The listing builds one solid part. Answer for the finished solid, in the listing's coordinates (mm). Face numbers are marked on the shaded views. A direction names the side the tool comes from. Coordinates: 2 decimals unless noted, no trailing zeros. Order: outer loops, then holes, each group sorted by start corner. A loop starts at its lowest first (then second) coordinate and runs counter-clockwise, first axis right, second up. Notation, with made-up numbers: (36.25, 36) -> (88.25, 36) arc R18 cw to (88.25, 70) -> close; hole circle Ø11 at (-31, -29.5). An arc over 180 degrees is marked (long way). Answer in a Markdown table with one row per item.
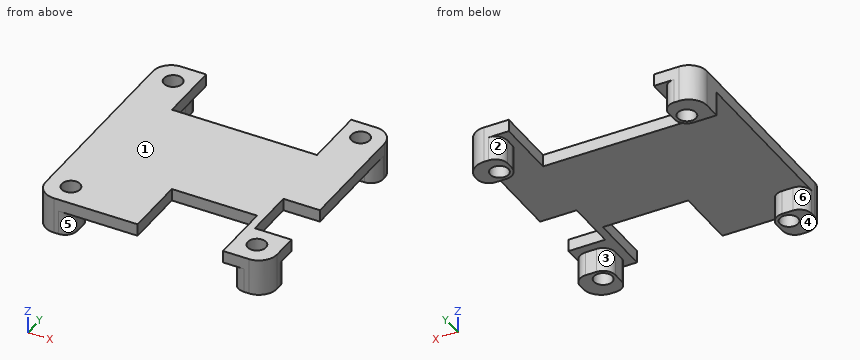
```python
from build123d import *

# Parameters (mm, degrees)
F0_R        = 1.5
F1_DEPTH    = 2
F2_DEPTH    = 4
F3_T1_DEPTH = 9
F4_T1_DEPTH = 9
F4_T3_DEPTH = 8.8612846748


# Not quite as in the source:
# - a fillet or chamfer that OpenCascade refuses, or shapes differently, is made with other operations: its cross-section is extruded or revolved along the edge and cut away or added


with BuildPart() as f1:
    # F0 (on Top) → F1 (new body)
    with BuildSketch(Plane.XY):
        with BuildLine():
            Line((11.75, -19), (13.2, -19))
            Line((13.2, -19), (13.2, -15.25))
            ThreePointArc((13.2, -15.25), (13.8004310986, -13.8004310986), (15.25, -13.2))
            Line((15.25, -13.2), (19, -13.2))
            Line((19, -13.2), (19, -11.75))
            Line((19, -11.75), (13, -11.75))
            Line((13, -11.75), (13, -3.25))
            Line((13, -3.25), (19, -3.25))
            Line((19, -3.25), (19, 13.6544716179))
            Line((19, 13.6544716179), (15.25, 13.6544716179))
            ThreePointArc((15.25, 13.6544716179), (13.8004310986, 14.2549027165), (13.2, 15.7044716179))
            Line((13.2, 15.7044716179), (13.2, 19))
            Line((13.2, 19), (11.9, 19))
            Line((11.9, 19), (11.9, 8.8))
            Line((11.9, 8.8), (0, 8.8))
            Line((0, 8.8), (-11.9, 8.8))
            Line((-11.9, 8.8), (-11.9, 19))
            Line((-11.9, 19), (-13.2, 19))
            Line((-13.2, 19), (-13.2, 15.25))
            ThreePointArc((-13.2, 15.25), (-13.8004310986, 13.8004310986), (-15.25, 13.2))
            Line((-15.25, 13.2), (-19, 13.2))
            Line((-19, 13.2), (-19, -13.2))
            Line((-19, -13.2), (-15.25, -13.2))
            ThreePointArc((-15.25, -13.2), (-13.7801859172, -13.8209630649), (-13.2008111101, -15.3076618908))
            Line((-13.2008111101, -15.3076618908), (-13.304709388, -19))
            Line((-13.304709388, -19), (-2.25, -19))
            Line((-2.25, -19), (-2.25, -8.8))
            Line((-2.25, -8.8), (11.75, -8.8))
            Line((11.75, -8.8), (11.75, -19))
        make_face()
        with BuildLine():
            Line((-19, 16), (-19, 13.2))
            Line((-19, 13.2), (-15.25, 13.2))
            ThreePointArc((-15.25, 13.2), (-13.8004310986, 13.8004310986), (-13.2, 15.25))
            Line((-13.2, 15.25), (-13.2, 19))
            Line((-13.2, 19), (-16, 19))
            ThreePointArc((-16, 19), (-18.1213203436, 18.1213203436), (-19, 16))
        make_face()
        with Locations((-15.25, 15.25)):
            Circle(F0_R, mode=Mode.SUBTRACT)
        with BuildLine():
            Line((15.25, 13.6544716179), (19, 13.6544716179))
            Line((19, 13.6544716179), (19, 16))
            ThreePointArc((19, 16), (18.1213203436, 18.1213203436), (16, 19))
            Line((16, 19), (13.2, 19))
            Line((13.2, 19), (13.2, 15.7044716179))
            ThreePointArc((13.2, 15.7044716179), (13.8004310986, 14.2549027165), (15.25, 13.6544716179))
        make_face()
        with Locations((15.25, 15.7044716179)):
            Circle(F0_R, mode=Mode.SUBTRACT)
        with BuildLine():
            Line((13.2, -19), (16, -19))
            ThreePointArc((16, -19), (18.1213203436, -18.1213203436), (19, -16))
            Line((19, -16), (19, -13.2))
            Line((19, -13.2), (15.25, -13.2))
            ThreePointArc((15.25, -13.2), (13.8004310986, -13.8004310986), (13.2, -15.25))
            Line((13.2, -15.25), (13.2, -19))
        make_face()
        with Locations((15.25, -15.25)):
            Circle(F0_R, mode=Mode.SUBTRACT)
        with BuildLine():
            Line((-16, -19), (-13.304709388, -19))
            Line((-13.304709388, -19), (-13.2008111101, -15.3076618908))
            ThreePointArc((-13.2008111101, -15.3076618908), (-13.7801859172, -13.8209630649), (-15.25, -13.2))
            Line((-15.25, -13.2), (-19, -13.2))
            Line((-19, -13.2), (-19, -16))
            ThreePointArc((-19, -16), (-18.1213203436, -18.1213203436), (-16, -19))
        make_face()
        with Locations((-15.25, -15.25)):
            Circle(F0_R, mode=Mode.SUBTRACT)
    extrude(amount=F1_DEPTH)

    # F0 (on Top) → F2 (join)
    with BuildSketch(Plane.XY):
        with BuildLine():
            Line((-16, -19), (-13.304709388, -19))
            Line((-13.304709388, -19), (-13.2008111101, -15.3076618908))
            ThreePointArc((-13.2008111101, -15.3076618908), (-13.7801859172, -13.8209630649), (-15.25, -13.2))
            Line((-15.25, -13.2), (-19, -13.2))
            Line((-19, -13.2), (-19, -16))
            ThreePointArc((-19, -16), (-18.1213203436, -18.1213203436), (-16, -19))
        make_face()
        with Locations((-15.25, -15.25)):
            Circle(F0_R, mode=Mode.SUBTRACT)
        with BuildLine():
            Line((13.2, -19), (16, -19))
            ThreePointArc((16, -19), (18.1213203436, -18.1213203436), (19, -16))
            Line((19, -16), (19, -13.2))
            Line((19, -13.2), (15.25, -13.2))
            ThreePointArc((15.25, -13.2), (13.8004310986, -13.8004310986), (13.2, -15.25))
            Line((13.2, -15.25), (13.2, -19))
        make_face()
        with Locations((15.25, -15.25)):
            Circle(F0_R, mode=Mode.SUBTRACT)
        with BuildLine():
            Line((15.25, 13.6544716179), (19, 13.6544716179))
            Line((19, 13.6544716179), (19, 16))
            ThreePointArc((19, 16), (18.1213203436, 18.1213203436), (16, 19))
            Line((16, 19), (13.2, 19))
            Line((13.2, 19), (13.2, 15.7044716179))
            ThreePointArc((13.2, 15.7044716179), (13.8004310986, 14.2549027165), (15.25, 13.6544716179))
        make_face()
        with Locations((15.25, 15.7044716179)):
            Circle(F0_R, mode=Mode.SUBTRACT)
        with BuildLine():
            Line((-19, 16), (-19, 13.2))
            Line((-19, 13.2), (-15.25, 13.2))
            ThreePointArc((-15.25, 13.2), (-13.8004310986, 13.8004310986), (-13.2, 15.25))
            Line((-13.2, 15.25), (-13.2, 19))
            Line((-13.2, 19), (-16, 19))
            ThreePointArc((-16, 19), (-18.1213203436, 18.1213203436), (-19, 16))
        make_face()
        with Locations((-15.25, 15.25)):
            Circle(F0_R, mode=Mode.SUBTRACT)
    extrude(amount=-F2_DEPTH)

    # F3: fillet of radius 2 on 1 edges, made by hand

    # F3_s2 → F3_t1 (cut)
    with BuildSketch(Plane.XY.offset(-9)):
        with BuildLine():
            ThreePointArc((-13.2, 17), (-13.7857864376, 18.4142135624), (-15.2, 19))
            Line((-15.2, 19), (-13.2, 19))
            Line((-13.2, 19), (-13.2, 17))
        make_face()
    extrude(amount=F3_T1_DEPTH, mode=Mode.SUBTRACT)

    # F4: fillet of radius 2 on 6 edges, made by hand

    # F4_s2 → F4_t1 (cut)
    with BuildSketch(Plane.XY.offset(-9)):
        with BuildLine():
            ThreePointArc((13.2, 17), (13.7857864376, 18.4142135624), (15.2, 19))
            Line((15.2, 19), (13.2, 19))
            Line((13.2, 19), (13.2, 17))
        make_face()
        with BuildLine():
            ThreePointArc((17, 13.6544716179), (18.4142135624, 14.2402580556), (19, 15.6544716179))
            Line((19, 15.6544716179), (19, 13.6544716179))
            Line((19, 13.6544716179), (17, 13.6544716179))
        make_face()
        with BuildLine():
            ThreePointArc((17, -13.2), (18.4142135624, -13.7857864376), (19, -15.2))
            Line((19, -15.2), (19, -13.2))
            Line((19, -13.2), (17, -13.2))
        make_face()
        with BuildLine():
            ThreePointArc((13.2, -17), (13.7857864376, -18.4142135624), (15.2, -19))
            Line((15.2, -19), (13.2, -19))
            Line((13.2, -19), (13.2, -17))
        make_face()
        with BuildLine():
            ThreePointArc((-17, -13.2), (-18.4142135624, -13.7857864376), (-19, -15.2))
            Line((-19, -15.2), (-19, -13.2))
            Line((-19, -13.2), (-17, -13.2))
        make_face()
    extrude(amount=F4_T1_DEPTH, mode=Mode.SUBTRACT)

    # F4_s4 → F4_t3 (cut)
    with BuildSketch(Plane.XY.offset(-8.8612846748)):
        with BuildLine():
            ThreePointArc((-13.2500145849, -17.0562555032), (-13.8550408822, -18.4339649588), (-15.249223258, -19))
            Line((-15.249223258, -19), (-13.304709388, -19))
            Line((-13.304709388, -19), (-13.2500145849, -17.0562555032))
        make_face()
    extrude(amount=F4_T3_DEPTH, mode=Mode.SUBTRACT)


solid = f1.part
```
(1) A cutting plane is placed at A-A, the plane z = -1.15. Count the separate pieces of the cut face and the enclosed holes in it, then the cut area to 3 significant figures.
Check values:
| item | result |
|---|---|
| separate pieces | 4 |
| enclosed holes | 4 |
| area | 86.2 mm² |
(2) A cutting plane is placed at C-C, the plane x = 4. Determine the outline of the cut face in (y, z).
Check values:
| item | result |
|---|---|
| outline | (-8.8, 0) -> (8.8, 0) -> (8.8, 2) -> (-8.8, 2) -> close |
(3) Find the intervals of material crossed by line 1 along Y through (x, z) = (15.25, 0.75); line 2 along Y through (x, z) = (15.25, -1.6); line 3 along Z through (x, y) = (16.5, -2.5), in increasing order. Write a range as from..to.
Check values:
| item | result |
|---|---|
| line 1 | -19..-16.75, -13.75..-11.75, -3.25..14.2, 17.2..19 |
| line 2 | -19..-16.75, -13.75..-13.2, 13.65..14.2, 17.2..19 |
| line 3 | 0..2 |
(4) Flat-ended cylindrical pins translate along their axes: pin 1 (2 mm diameter, centred on x = 5, z = 0.5, fed in from -Y); pin 2 (0.6 mm diameter, centred on x = 16.5, z = 0.5, fed in from +Y); pin 3 (1.8 mm diameter, centred on x = -15.25, y = 15.25, fed in from +Z); pin 4 (12 mm diameter, centred on x = -7.5, y = 2.5, fed in from -Z). Find the tip coordinate at first contact, or state that the pin passes through.
Check values:
| item | result |
|---|---|
| pin 1 | y = -8.8 |
| pin 2 | y = 18.99 |
| pin 3 | through |
| pin 4 | z = 0 |
(5) A cutting plane is placed at B-B, the plane y = -2. Determine the outline of the cut face in (x, z).
Check values:
| item | result |
|---|---|
| outline | (-19, 0) -> (19, 0) -> (19, 2) -> (-19, 2) -> close |
(6) Which of the six approach directions +Z, -Z, +X, -X, +Y, -Y give full straight-line access (tool end or side, diameter ignored) to the marked faces 4, 5 and 6?
Check values:
| item | result |
|---|---|
| face 4 | -Z, +X, -X, +Y, -Y |
| face 5 | -Z, -Y |
| face 6 | -Z, -X |
(7) For a pull along Y with two mould halves and no side action, classify the marked faces 1, 2 and 3 as released by +Y, released by -Y, zero draft, split by the parting line, or undercut.
Check values:
| item | result |
|---|---|
| face 1 | zero draft |
| face 2 | released by +Y |
| face 3 | undercut |
